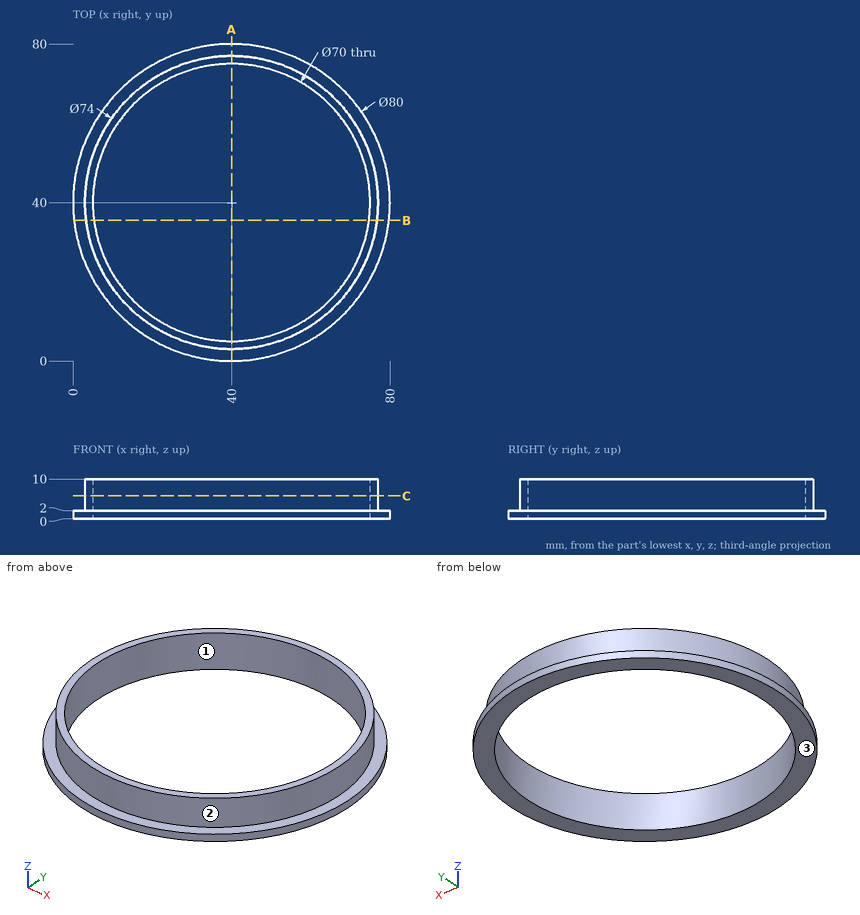
Geometry check sheet. Reference: drawing and pictorial views, mm from the part's lowest x, y, z. Give positions to 0.01 mm unless a question says otherwise; leave off trailing zeros. Loops run counter-clockwise (first coordinate to the right, second up) from the corner with the lowest first, then second, coordinate; pieces in that order, holes last. Notation, with made-up numbers: (69, 60.5) - (76, 60.5) arc R12 cw to (76, 68.5) - close; hole circle Ø5 at (-16, -39.75). An arc over 180 degrees is marked (long way). One line per question, with ' | ' between items. Start each with the question number.
1. Cross-section at A-A, the plane x = 40. Enter the section's corners in (y, z), plus the area to 3 significant figures.
2. Cross-section at B-B, the plane y = 35.5. Enter the section's corners in (x, z), plus the area to 3 significant figures.
3. Gauge pin test, flat ends, axial feed: pin 1 Ø3 at (y, z) = (34, 7) entering from -X; pin 2 Ø3 at (x, z) = (34.5, 6.5) entering from -Y; pin 3 Ø6 at (y, z) = (44.5, 6.5) entering from -X. Record the tip position at first contact, or that the pin passes through.
4. Cross-section at C-C, the plane z = 5.75. Enter the section's corners in (x, y).
5. Material ranges on line 1 along Y through (x, z) = (40, 3); line 2 along X through (y, z) = (30.5, 5.5); line 3 along X through (y, z) = (14, 8.25), recorded low to high. Write a range as [from, to].
6. Draft check along X on the marked faces 1, 2 and 3. Enter one of: released by +X, released by -X, zero draft, split by the parting line, or undercut.
Check result:
1) outline: (0, 0) - (5, 0) - (5, 10) - (3, 10) - (3, 2) - (0, 2) - close; (75, 0) - (80, 0) - (80, 2) - (77, 2) - (77, 10) - (75, 10) - close | area: 52.0 mm2
2) outline: (0.25, 0) - (5.29, 0) - (5.29, 10) - (3.27, 10) - (3.27, 2) - (0.25, 2) - close; (74.71, 0) - (79.75, 0) - (79.75, 2) - (76.73, 2) - (76.73, 10) - (74.71, 10) - close | area: 52.4 mm2
3) pin 1: stops at x = 3.27 | pin 2: stops at y = 3.22 | pin 3: stops at x = 3.03
4) outline: circle Ø74 at (40, 40); hole circle Ø70 at (40, 40)
5) line 1: y = [3, 5], [75, 77] | line 2: x = [4.24, 6.31], [73.69, 75.76] | line 3: x = [13.68, 16.57], [63.43, 66.32]
6) face 1: undercut | face 2: split by the parting line | face 3: zero draft
